The model under review builds one solid part; all positions refer to its coordinate system, in mm. A direction names the side the tool comes from. Round coordinates to 2 decimals unless told otherwise and drop trailing zeros. Order: outer loops, then holes, each group sorted by start corner. A loop starts at its lowest first (then second) coordinate and runs counter-clockwise, first axis right, second up. Notation, with made-up numbers: (17, -24.75) -> (27, -24.75) arc R27 cw to (27, 3.25) -> close; hole circle Ø9 at (-8, 87.25). An arc over 180 degrees is marked (long way). Return JSON: item names as keys, results as strings. Group by question number.
Autodesk Inventor part; units mm, degrees
ref_plane "YZ Plane" through (0, 0, 0) normal (1, 0, 0) x (0, 1, 0)
ref_plane "XZ Plane" through (0, 0, 0) normal (0, 1, 0) x (-1, 0, 0)
ref_plane "XY Plane" through (0, 0, 0) normal (0, 0, 1) x (1, 0, 0)
sketch "Sketch1" plane through (0, 0, 0) normal (1, 0, 0) x (0, 1, 0)
  line L0 (0, 0) -> (181, 0)
  line L1 (181, 0) -> (181, -9)
  line L2 (0, -9) -> (0, 0)
  line L3 (15.1, -9) -> (15.1, -4)
  line L4 (15.1, -4) -> (5, -4)
  line L5 (5, -4) -> (5, -9)
  line L6 (165.9, -9) -> (165.9, -4)
  line L7 (165.9, -4) -> (176, -4)
  line L8 (176, -4) -> (176, -9)
  line L9 (5, -9) -> (0, -9)
  line L10 (181, -9) -> (176, -9)
  line L11 (165.9, -9) -> (15.1, -9)
  dimension "d0" = 181
  dimension "d1" = 10.1
  dimension "d3" = 10.1
  dimension "d5" = 5
  dimension "d7" = 5
  dimension "d8" = 5
  dimension "d11" = 9
  dimension "d12" = 171
  dimension "d17" = 9
  dimension "d18" = 9
extrude "Extrusion1" add sketch "Sketch1" along normal blind 9.9
fillet "Fillet1" radius 0.5 4 edges at (4.95, 176, -4) (4.95, 165.9, -4) (4.95, 15.1, -4) (4.95, 5, -4)
chamfer "Chamfer1" distance 0.5 angle 45 40 edges at (9.9, 90.5, 0) (9.9, 90.5, -9) (9.9, 15.1, -6.75) (9.9, 14.9536, -4.1464) (9.9, 10.05, -4) (9.9, 5.1464, -4.1464) (9.9, 5, -6.75) (9.9, 0, -4.5) (9.9, 2.5, -9) (4.95, 0, -9) (0, 0, -4.5) (4.95, 0, 0) (0, 90.5, 0) (9.9, 176, -6.75) (9.9, 175.8536, -4.1464) (9.9, 170.95, -4) (9.9, 166.0464, -4.1464) (9.9, 165.9, -6.75) (9.9, 178.5, -9) (9.9, 181, -4.5) (0, 181, -4.5) (0, 178.5, -9) (4.95, 176, -9) (4.95, 181, -9) (4.95, 181, 0) (4.95, 15.1, -9) (4.95, 165.9, -9) (0, 170.95, -4) (0, 175.8536, -4.1464) (0, 176, -6.75) (0, 166.0464, -4.1464) (0, 165.9, -6.75) (0, 90.5, -9) (0, 15.1, -6.75) (0, 14.9536, -4.1464) (0, 10.05, -4) (0, 5.1464, -4.1464) (0, 5, -6.75) (0, 2.5, -9) (4.95, 5, -9)
equation "\"d5\" = -0.5 * d12 + 0.5 * d0"
equation "\"d17\" = d11"
equation "\"d18\" = d17"
properties part number "LegsStabilizer"
Item 1: Wall thickness on line 1 along Y through (x, z) = (5, -4.75); line 2 along Z through (x, y) = (0.75, 166.5); line 3 along Z through (x, y) = (9.5, 23.5): over which ranges is each line inside the solid? List them lowest first.
Item 2: Consider section B-B on y = 11. State the section outline as (x, z) points, plus the area to 3 significant figures.
Item 3: Consider section A-A on x = 6.25. State the section outline as (y, z) points, plus the area to 3 significant figures.
Item 4: For faces 1 (the face through (5, 10, -4)), 2 (the face through (5, 89, 0)), list the 3-axis set-ups (+Z, -Z, +X, -X, +Y, -Y) from which the entire face can be reached by the end or side of a thin tool; tool diameter is ignored.
Values:
{
 "1": {"line 1": "0 to 5, 15.1 to 165.9, 176 to 181", "line 2": "-4 to 0", "line 3": "-8.9 to -0.1"},
 "2": {"outline": "(0, -3.5) -> (0.5, -4) -> (9.4, -4) -> (9.9, -3.5) -> (9.9, -0.5) -> (9.4, 0) -> (0.5, 0) -> (0, -0.5) -> close", "area": "39.1 mm^2"},
 "3": {"outline": "(0, -8.5) -> (0.5, -9) -> (4.5, -9) -> (5, -8.5) -> (5, -4.5) arc R0.5 cw to (5.5, -4) -> (14.6, -4) arc R0.5 cw to (15.1, -4.5) -> (15.1, -8.5) -> (15.6, -9) -> (165.4, -9) -> (165.9, -8.5) -> (165.9, -4.5) arc R0.5 cw to (166.4, -4) -> (175.5, -4) arc R0.5 cw to (176, -4.5) -> (176, -8.5) -> (176.5, -9) -> (180.5, -9) -> (181, -8.5) -> (181, -0.5) -> (180.5, 0) -> (0.5, 0) -> (0, -0.5) -> close", "area": "1,530 mm^2"},
 "4": {"face 1": "-Z, +X, -X", "face 2": "+Z, +X, -X, +Y, -Y"}
}
